from build123d import *

# Parameters (mm, degrees)
SKETCH002_R       = 1.6
EXTRUDE002_DEPTH  = 2.5
SKETCH003_R       = 1.6
EXTRUDE003_DEPTH  = 2.5
SKETCH004_R       = 1.6
EXTRUDE004_DEPTH  = 2.5
SKETCH001_R       = 1.6
EXTRUDE001_DEPTH  = 2.5
SKETCH_R          = 1.6
EXTRUDE_DEPTH     = 10
CYLINDER007_R     = 1.6
CYLINDER007_DEPTH = 10
CYLINDER006_R     = 1.6
CYLINDER006_DEPTH = 10
CYLINDER005_R     = 1.6
CYLINDER005_DEPTH = 10
CYLINDER004_R     = 1.6
CYLINDER004_DEPTH = 10
BOX001_W          = 104
BOX001_H          = 62
BOX001_DEPTH      = 4


with BuildPart() as nylon_nut_cutout001:
    # Sketch002 → Extrude002 (new body)
    with BuildSketch(Plane.XY):
        Polygon((3.2, 0), (1.6, 2.771281), (-1.6, 2.771281), (-3.2, 0), (-1.6, -2.771281), (1.6, -2.771281), align=None)
        Circle(SKETCH002_R, mode=Mode.SUBTRACT)
    extrude(amount=EXTRUDE002_DEPTH)


with BuildPart() as nylon_nut_cutout001_1:
    # Extrude002 placement: moved
    add(nylon_nut_cutout001.part.moved(Location((-72.8, 6.2, 0))))


with BuildPart() as nylon_nut_cutout002:
    # Sketch003 → Extrude003 (new body)
    with BuildSketch(Plane.XY):
        Polygon((3.2, 0), (1.6, 2.771281), (-1.6, 2.771281), (-3.2, 0), (-1.6, -2.771281), (1.6, -2.771281), align=None)
        Circle(SKETCH003_R, mode=Mode.SUBTRACT)
    extrude(amount=EXTRUDE003_DEPTH)


with BuildPart() as nylon_nut_cutout002_1:
    # Extrude003 placement: moved
    add(nylon_nut_cutout002.part.moved(Location((-72.8, 55.8, 0))))


with BuildPart() as nylon_nut_cutout003:
    # Sketch004 → Extrude004 (new body)
    with BuildSketch(Plane.XY):
        Polygon((3.2, 0), (1.6, 2.771281), (-1.6, 2.771281), (-3.2, 0), (-1.6, -2.771281), (1.6, -2.771281), align=None)
        Circle(SKETCH004_R, mode=Mode.SUBTRACT)
    extrude(amount=EXTRUDE004_DEPTH)


with BuildPart() as nylon_nut_cutout003_1:
    # Extrude004 placement: moved
    add(nylon_nut_cutout003.part.moved(Location((-14.2, 55.8, 0))))


with BuildPart() as nylon_nut_cutout:
    # Sketch001 → Extrude001 (new body)
    with BuildSketch(Plane.XY):
        Polygon((3.2, 0), (1.6, 2.771281), (-1.6, 2.771281), (-3.2, 0), (-1.6, -2.771281), (1.6, -2.771281), align=None)
        Circle(SKETCH001_R, mode=Mode.SUBTRACT)
    extrude(amount=EXTRUDE001_DEPTH)


with BuildPart() as nylon_nut_cutout_1:
    # Extrude001 placement: moved
    add(nylon_nut_cutout.part.moved(Location((-14.2, 6.2, 0))))


with BuildPart() as extrude_body:
    # Sketch → Extrude (new body)
    with BuildSketch(Plane.XY):
        with Locations((-72.8, 55.8)):
            Circle(SKETCH_R)
        with Locations((-14.2, 55.8)):
            Circle(SKETCH_R)
        with Locations((-14.2, 6.2)):
            Circle(SKETCH_R)
        with Locations((-72.8, 6.2)):
            Circle(SKETCH_R)
    extrude(amount=EXTRUDE_DEPTH)


with BuildPart() as mount_point003:
    # Cylinder007 → Cylinder007 (new body)
    with BuildSketch(Plane(origin=(-3.1, 58.9, 0), x_dir=(1, 0, 0), z_dir=(0, 0, 1))):
        Circle(CYLINDER007_R)
    extrude(amount=CYLINDER007_DEPTH)


with BuildPart() as mount_point002:
    # Cylinder006 → Cylinder006 (new body)
    with BuildSketch(Plane(origin=(-100.9, 58.9, 0), x_dir=(1, 0, 0), z_dir=(0, 0, 1))):
        Circle(CYLINDER006_R)
    extrude(amount=CYLINDER006_DEPTH)


with BuildPart() as mount_point001:
    # Cylinder005 → Cylinder005 (new body)
    with BuildSketch(Plane(origin=(-100.9, 3.1, 0), x_dir=(1, 0, 0), z_dir=(0, 0, 1))):
        Circle(CYLINDER005_R)
    extrude(amount=CYLINDER005_DEPTH)


with BuildPart() as mount_point:
    # Cylinder004 → Cylinder004 (new body)
    with BuildSketch(Plane(origin=(-2.6, 3.1, 0), x_dir=(1, 0, 0), z_dir=(0, 0, 1))):
        Circle(CYLINDER004_R)
    extrude(amount=CYLINDER004_DEPTH)


with BuildPart() as obj1:
    # Box001 → Box001 (new body)
    with BuildSketch(Plane(origin=(-104, 0, 0), x_dir=(1, 0, 0), z_dir=(0, 0, 1))):
        with Locations((52, 31)):
            Rectangle(BOX001_W, BOX001_H)
    extrude(amount=BOX001_DEPTH)

    # Cut005: cut Mount Point
    add(mount_point.part, mode=Mode.SUBTRACT)

    # Cut006: cut Mount Point001
    add(mount_point001.part, mode=Mode.SUBTRACT)

    # Cut007: cut Mount Point002
    add(mount_point002.part, mode=Mode.SUBTRACT)

    # Cut008: cut Mount Point003
    add(mount_point003.part, mode=Mode.SUBTRACT)

    # Cut: cut Extrude body
    add(extrude_body.part, mode=Mode.SUBTRACT)

    # Cut009: cut Nylon Nut Cutout
    add(nylon_nut_cutout_1.part, mode=Mode.SUBTRACT)

    # Cut010: cut Nylon Nut Cutout003
    add(nylon_nut_cutout003_1.part, mode=Mode.SUBTRACT)

    # Cut011: cut Nylon Nut Cutout002
    add(nylon_nut_cutout002_1.part, mode=Mode.SUBTRACT)

    # Cut012: cut Nylon Nut Cutout001
    add(nylon_nut_cutout001_1.part, mode=Mode.SUBTRACT)


solid = obj1.part
Model file for the job. Use its own axes, mm. A direction names the side the tool comes from. Round coordinates to 2 decimals unless told otherwise and drop trailing zeros. Loops run counter-clockwise (first coordinate to the right, second up) from the corner with the lowest first, then second, coordinate; pieces in that order, holes last. Notation, with made-up numbers: (79.25, 12.5) -> (108.25, 12.5) arc R20 ccw to (108.25, 39.5) -> close; hole circle Ø7 at (-20, 36). An arc over 180 degrees is marked (long way). Answer as CSV lines item,"result". Start each with the question number.
1) Tool access for faces 4 (the face through (-74.4, 6.27, 3.24)), 5 (the face through (-70.39, 7.57, 1.23)): list every direction of +Z, -Z, +X, -X, +Y, -Y with a clear straight run to the whole face (end or side of a thin tool).
2) Probe line 1 along X through (y, z) = (3.1, 2.6); line 2 along X through (y, z) = (58.9, 3.25); line 3 along Y through (x, z) = (-72.8, 3.7). List the from-to ranges inside material, lowest first.
3) Pin check, flat tip, straight feed: P1, Ø3, axis at x = -13.5, y = 7, coming from the -Z side. Stop position of the tip, or through.
4) Slice it at A-A (x = -100.9). List the corners of the cut face in (y, z), plus the area to 3 significant figures.
5) Mould opens along Y. For faces 1 (the face through (-74.4, 55.87, 3.24)), 2 (the face through (0, 31, 2)), 3 (the face through (-53, 0, 2)) say: +Y half, -Y half, draft (parallel to the pull), parting line (faces both ways), or undercut.
6) Slice it at B-B (z = 1.9). State how many separate pieces and enclosed holes the cut face has, plus the area to 3 significant figures.
Filled in:
1,face 4,"+Z, -Z"
1,face 5,"-Z"
2,line 1,"x = -104 to -102.5, -99.3 to -4.2, -1 to 0"
2,line 2,"x = -104 to -102.5, -99.3 to -4.7, -1.5 to 0"
2,line 3,"y = 0 to 4.6, 7.8 to 54.2, 57.4 to 62"
3,P1,"stops at z = 2.5"
4,outline,"(0, 0) -> (1.5, 0) -> (1.5, 4) -> (0, 4) -> close; (4.7, 0) -> (57.3, 0) -> (57.3, 4) -> (4.7, 4) -> close; (60.5, 0) -> (62, 0) -> (62, 4) -> (60.5, 4) -> close"
4,area,"222 mm2"
5,face 1,"undercut"
5,face 2,"draft"
5,face 3,"-Y half"
6,separate pieces,"1"
6,enclosed holes,"8"
6,area,"6,310 mm2"
